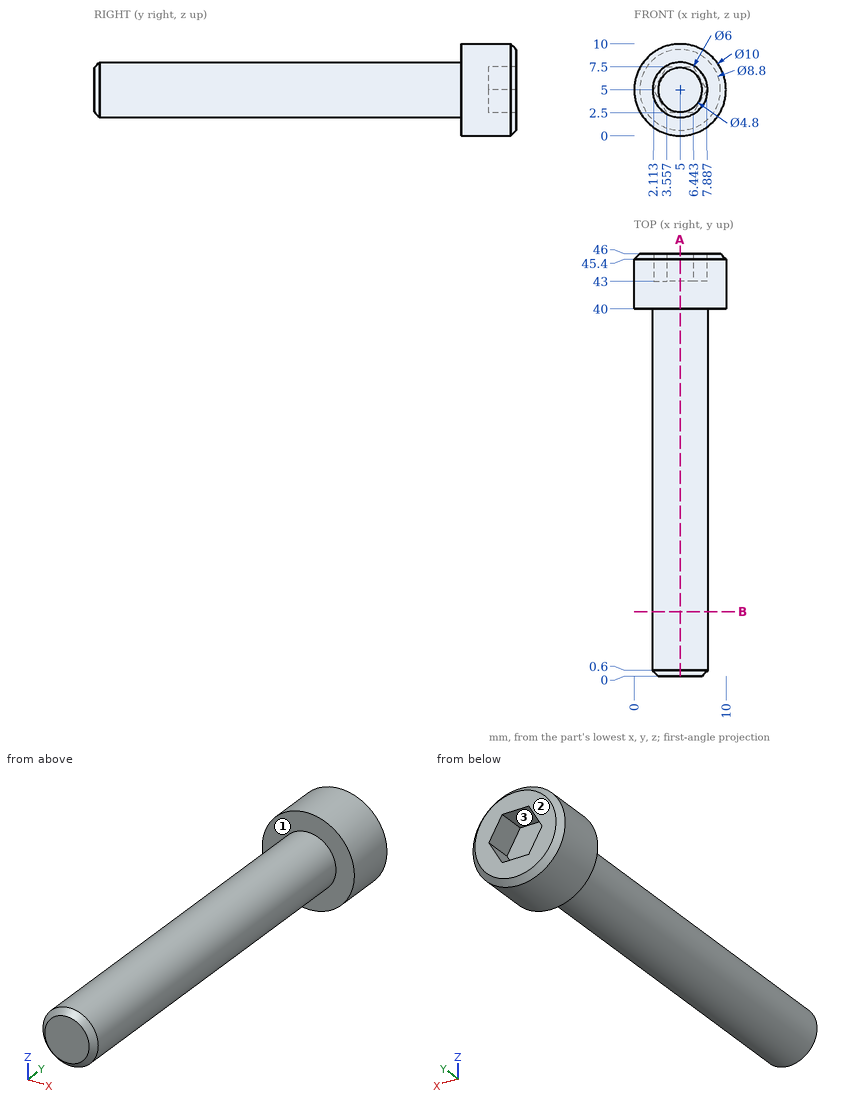
Answer from the drawing. Dimensions are ordinates in mm from the lowest x, y and z of the part. A direction names the side the tool comes from. Round coordinates to 2 decimals unless told otherwise and drop trailing zeros. Write each loop counter-clockwise with the first axis right and the second up, starting at its lowest first coordinate (ties: lowest second). Pieces come first, ordered by that corner, then holes. Notation, with made-up numbers: M 6.25,89.5 L 50.25,89.5 A24 ccw 50.25,124.5 Z; hole C 27.5,-39.5 d9. An arc over 180 degrees is marked long. Write each question's results on one line, items separated by ' | '. Start each with the question number.
Item 1: Flat-ended cylindrical pins translate along their axes: pin 1 Ø1.5 at (x, z) = (4.5, 4) entering from +Y; pin 2 Ø2 at (x, z) = (2.5, 3) entering from -Y; pin 3 Ø6 at (y, z) = (40.5, 1.5) entering from -X (1 decimal); pin 4 Ø4 at (x, y) = (8, 30) entering from -Z. Find the tip coordinate at first contact, or state that the pin passes through.
Item 2: For the marked faces 1, 2 and 3, determine the directions among +Z, -Z, +X, -X, +Y, -Y from which every point of the face is accessible in a straight line to the end or side of a thin tool.
Item 3: A cutting plane is placed at B-B on y = 7. Write down the section's boundary in (x, z).
Item 4: Straight lines are drawn through the part: L1, parallel to Y at x = 1.75, z = 4.75; L2, parallel to Y at x = 3.75, z = 4; L3, parallel to Z at x = 5, y = 32. For each, find the intervals that lie inside material, in ascending order. Write a range as [from, to].
Item 5: A cutting plane is placed at A-A on x = 5. Write down the section's boundary in (y, z), and give its area (3 significant figures).
Check sheet entries:
1) pin 1: y = 43 | pin 2: y = 0 | pin 3: x = 0 | pin 4: z = 2.17
2) face 1: -Y | face 2: +Z, -Z, +X, -X, +Y | face 3: +Y
3) outline: C 5,5 d6
4) L1: [40, 46] | L2: [0, 43] | L3: [2, 8]
5) outline: M 0,2.6 L 0.6,2 L 40,2 L 40,0 L 45.4,0 L 46,0.6 L 46,2.5 L 43,2.5 L 43,7.5 L 46,7.5 L 46,9.4 L 45.4,10 L 40,10 L 40,8 L 0.6,8 L 0,7.4 Z | area: 284 mm²
